Here's the drawing with two shaded views (mm, measured from the low corner). I have some questions. A direction names the side the tool comes from. Round coordinates to 2 decimals unless told otherwise and drop trailing zeros. Order: outer loops, then holes, each group sorted by start corner. A loop starts at its lowest first (then second) coordinate and runs counter-clockwise, first axis right, second up.
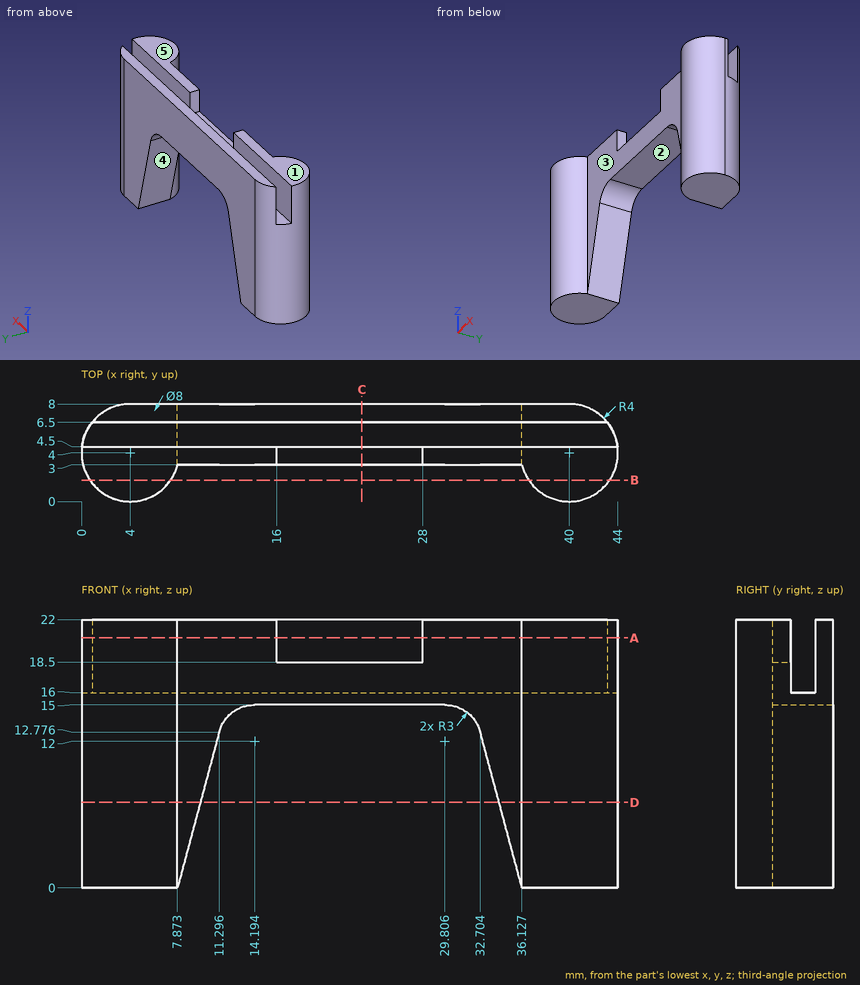
Q1. Imagine slicing it at D-D, the plane z = 7. Please give me the cut outline in (x, y), then the cut area to 3 significant figures.
Q2. We'd pull the mould along X, two halves only. Please class the marked faces 1 and 2: released by +X, released by -X, zero draft, split by the parting line, or undercut.
Q3. Imagine slicing it at A-A, the plane z = 20.5. Please give me the cut outline in (x, y).
Q4. For the marked faces 3, 4 and 5, which set-ups out of +Z, -Z, +X, -X, +Y, -Y let a thin tool reach every point of the face, with its end or its side?
Q5. For P1, Ø12, axis at x = 12.5, z = 6.5, coming from the -Y side; P2, Ø6.5, axis at x = 24, z = 20.5, coming from the -Y side; P3, Ø3, axis at y = 2, z = 5, coming from the -X side, each with a flat end and sliding along its axis, tell me the tip position at first contact or that it passes through.
Q6. Imagine slicing it at C-C, the plane x = 23. Please give me the cut outline in (y, z).
Q7. I need wall thicknesses on L1, parallel to Y at x = 26, z = 17.75; L2, parallel to Z at x = 27, y = 5; L3, parallel to Y at x = 25, z = 18.75. Which ranges of each line are inside material? Lowest first, please.
Q8. Imagine slicing it at B-B, the plane y = 1.75. Please give me the cut outline in (x, z).
Filled in:
1. outline: (4, 8) arc R4 ccw (long way) to (7.87, 3) - (9.75, 3) - (9.75, 8) - close; (34.25, 3) - (36.13, 3) arc R4 ccw (long way) to (40, 8) - (34.25, 8) - close
1. area: 125 mm2
2. face 1: zero draft
2. face 2: undercut
3. outline: (0.03, 4.5) arc R4 ccw to (7.87, 3) - (16, 3) - (16, 4.5) - close; (0.88, 6.5) - (43.12, 6.5) arc R4 ccw to (40, 8) - (4, 8) arc R4 ccw to start; (28, 3) - (36.13, 3) arc R4 ccw to (43.97, 4.5) - (28, 4.5) - close
4. face 3: +Z, -Z, -Y
4. face 4: -Z, +Y, -Y
4. face 5: +Z, +X, -X, +Y, -Y
5. P1: stops at y = 0.88
5. P2: stops at y = 3
5. P3: stops at x = 0.03
6. outline: (3, 15) - (8, 15) - (8, 22) - (6.5, 22) - (6.5, 16) - (4.5, 16) - (4.5, 18.5) - (3, 18.5) - close
7. L1: y = 3 to 4.5, 6.5 to 8
7. L2: z = 15 to 16
7. L3: y = 6.5 to 8
8. outline: (0.69, 0) - (7.31, 0) - (7.31, 22) - (0.69, 22) - close; (36.69, 0) - (43.31, 0) - (43.31, 22) - (36.69, 22) - close
